Autodesk Inventor part; units mm, degrees
ref_plane "YZ Plane" through (0, 0, 0) normal (1, 0, 0) x (0, 1, 0)
ref_plane "XZ Plane" through (0, 0, 0) normal (0, 1, 0) x (-1, 0, 0)
ref_plane "XY Plane" through (0, 0, 0) normal (0, 0, 1) x (1, 0, 0)
sketch "Sketch1" plane through (0, 0, 0) normal (1, 0, 0) x (0, 1, 0)
  line L0 (-12.5, 15) -> (12.5, 15)
  line L1 (12.5, 15) -> (12.5, -15)
  line L2 (12.5, -15) -> (-12.5, -15)
  line L3 (-12.5, -15) -> (-12.5, 15)
  line L4 (-12.5, 15) -> (12.5, -15) construction
  line L5 (12.5, 15) -> (-12.5, -15) construction
  line L6 (0, -15) -> (0, -1.5)
  circle A0 centre (0, -1.5) radius 8
  point P0 (0, 0)
  dimension "d0" = 25
  dimension "d1" = 30
  dimension "d2" = 13.5
  dimension "d3" = 16
extrude "Extrusion1" add sketch "Sketch1" along normal blind 8
sketch "Sketch2" plane through (8, 0, 0) normal (1, 0, 0) x (0, 0, -1)
  line L0 (7.5, -1) -> (22.5, -1)
  line L1 (22.5, -1) -> (22.5, 1)
  line L2 (22.5, 1) -> (7.5, 1)
  line L3 (7.5, 1) -> (7.5, -1)
  line L4 (15, -12.5) -> (15, 12.5)
  line L5 (7.5, -1) -> (22.5, 1) construction
  line L6 (22.5, -1) -> (7.5, 1) construction
  point P0 (0, 0)
  point P1 (15, 0)
  dimension "d6" = 2
  dimension "d17" = 15
extrude "Extrusion2" cut sketch "Sketch2" against normal up to next
sketch "Sketch3" plane through (0, 12.5, 15) normal (0, 1, 0) x (1, 0, 0)
  line L0 (0, 0) -> (8, 0)
  line L1 (4, 0) -> (4, 5)
  circle A0 centre (4, 5) radius 2.1
  point P0 (0, 15)
  dimension "d9" = 5
  dimension "d10" = 4.2
extrude "Extrusion3" cut sketch "Sketch3" against normal up to next
sketch "Sketch4" plane through (0, 12.5, 15) normal (0, 1, 0) x (1, 0, 0)
  line L0 (0, 30) -> (8, 30)
  line L1 (4, 30) -> (4, 26.5)
  circle A0 centre (4, 26.5) radius 1.25
  point P0 (0, 15)
  dimension "d13" = 3.5
  dimension "d14" = 2.5
extrude "Extrusion4" cut sketch "Sketch4" against normal through all
fillet "Fillet1" radius 4 2 edges at (0, 0, 15) (8, 0, 15)
fillet "Fillet2" radius 2 2 edges at (0, 6.75, -15) (0, -6.75, -15)
properties part number "arm_grip" material "Nylon 6/6"
Can you work these out from the model? Positions are in its coordinate system, mm. A direction names the side the tool comes from. Give positions to 0.01 mm unless a question says otherwise; leave off trailing zeros. Order: outer loops, then holes, each group sorted by start corner. A loop starts at its lowest first (then second) coordinate and runs counter-clockwise, first axis right, second up. Notation, with made-up numbers: M 42.25,-15 L 75.25,-15 A7 cw 75.25,-10 Z; hole C 8,64 d2. An arc over 180 degrees is marked long. Write item = value, one per line. Start each with the question number.
Q1. We'd pull the mould along Z, two halves only. Please class faces 3 (the cylindrical face through (3.727, 0.175, 7.918)), 4 (the flat face through (5, 7, -15)), 5 (the flat face through (4, 12.5, 0)), 6 (the cylindrical face through (3.944, -0.338, 6.493)): pulls with the +Z half, pulls with the -Z half, needs draft (parallel to the pull), parting line crosses it, or undercut.
Q2. Suppose I cut it at C-C (z = -1.5). Write out the boundary of the cut face in (x, y), plus the area to 3 significant figures.
Q3. Suppose I cut it at A-A (z = -11.5). Write out the boundary of the cut face in (x, y), plus the area to 4 significant figures.
Q4. For faces 1 (the flat face through (4, 1, -13)), 2 (the cylindrical face through (6.797, 0.175, 13.859)), which set-ups out of +Z, -Z, +X, -X, +Y, -Y let a thin tool reach every point of the face, with its end or its side?
Q5. Will this pin go through, and if not, where does the flat tip stop? pin 1 Ø3 at (y, z) = (2, -8.5) entering from -X.
Q6. Suppose I cut it at B-B (y = -7). Count the separate pieces of the cut face and the enclosed holes in it, plus the area to 3 significant figures.
Q7. I need wall thicknesses on probe 1 along Z at (x, y) = (4, 11.5); probe 2 along Y at (x, z) = (5, -12.75); probe 3 along Y at (x, z) = (5.75, -1.5). Which ranges of each line are inside material? Lowest first, please. Write a range as [from, to].
Check result:
q1.face_3 = undercut
q1.face_4 = pulls with the -Z half
q1.face_5 = needs draft
q1.face_6 = undercut
q2.outline = M 0,-12.5 L 8,-12.5 L 8,-8 L 0,-8 Z; M 0,8 L 8,8 L 8,12.5 L 0,12.5 Z
q2.area = 72.0 mm2
q3.outline = M 0,-12.5 L 2.75,-12.5 L 2.75,-1 L 0,-1 Z; M 0,1 L 2.75,1 L 2.75,12.5 L 0,12.5 Z; M 5.25,-12.5 L 8,-12.5 L 8,-1 L 5.25,-1 Z; M 5.25,1 L 8,1 L 8,12.5 L 5.25,12.5 Z
q3.area = 126.5 mm2
q4.face_1 = -Z, +X, -X
q4.face_2 = +Z, +X, +Y, -Y
q5.pin_1 = 0
q6.separate_pieces = 2
q6.enclosed_holes = 2
q6.area = 152 mm2
q7.probe_1 = [-15, -12.75], [-10.25, 7.9], [12.1, 15]
q7.probe_2 = [-12.5, -1], [1, 12.5]
q7.probe_3 = [-12.5, -8], [8, 12.5]
